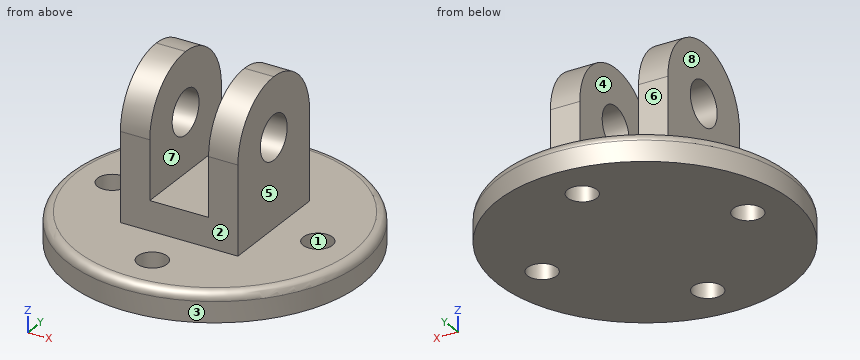
```python
from build123d import *

# Parameters (mm, degrees)
F0_R     = 63.5
F0_R_2   = 6.35
F1_DEPTH = 12.7
F2_R     = 3.81
F4_DEPTH = 25.4
F5_R     = 9.525
F6_DEPTH = 88.901


with BuildPart() as f1:
    # F0 (on Top) → F1 (new body)
    with BuildSketch(Plane.XY):
        Circle(F0_R)
        with Locations((0, -44.45)):
            Circle(F0_R_2, mode=Mode.SUBTRACT)
        with Locations((-44.45, 0)):
            Circle(F0_R_2, mode=Mode.SUBTRACT)
        with Locations((44.45, 0)):
            Circle(F0_R_2, mode=Mode.SUBTRACT)
        with Locations((0, 44.45)):
            Circle(F0_R_2, mode=Mode.SUBTRACT)
    extrude(amount=F1_DEPTH)

    # F2
    f2_edges = [f1.edges().sort_by_distance(p)[0] for p in [
        (-63.5, 0, 12.7),
    ]]
    fillet(f2_edges, radius=F2_R)

    # F3 (on Front) → F4 (join, symmetric)
    with BuildSketch(Plane.XZ):
        Polygon((-25.4, 76.2), (-25.4, 12.7), (25.4, 12.7), (25.4, 76.2), (12.7, 76.2), (12.7, 25.4), (-12.7, 25.4), (-12.7, 76.2), align=None)
    extrude(amount=F4_DEPTH, both=True)

    # F5 (on face) → F6 (cut, through all)
    with BuildSketch(Plane.YZ.offset(25.4)):
        with Locations((0, 50.8)):
            Circle(F5_R)
        with BuildLine():
            ThreePointArc((0, 76.2), (17.960512, 68.760512), (25.4, 50.8))
            Line((25.4, 50.8), (25.4, 76.2))
            Line((25.4, 76.2), (0, 76.2))
        make_face()
        with BuildLine():
            ThreePointArc((-25.4, 50.8), (-17.960512, 68.760512), (0, 76.2))
            Line((0, 76.2), (-25.4, 76.2))
            Line((-25.4, 76.2), (-25.4, 50.8))
        make_face()
    extrude(amount=-F6_DEPTH, mode=Mode.SUBTRACT)


solid = f1.part
```
Could you check a few things on this model? Use its own coordinates, in mm. Face numbers are marked on the shaded views. A direction names the side the tool comes from. Coordinates: 2 decimals unless noted, no trailing zeros. Loops run counter-clockwise (first coordinate to the right, second up) from the corner with the lowest first, then second, coordinate; pieces in that order, holes last. Notation, with made-up numbers: M 47,70.5 L 73,70.5 A18 cw 73,96.5 Z; hole C 24.25,-39.5 d10. An arc over 180 degrees is marked long. Put each result on its own line as item: value. Start each with the question number.
(1) Suppose I cut it at A-A on x = 0. Please give me the cut outline in (y, z), then the cut area to 3 significant figures.
(2) Thinking about a two-plate mould opening in X: for the marked faces 1, 2, 3 and 4, which applies, pulls with the +X half, pulls with the -X half, needs draft (parallel to the pull), parting line crosses it, or undercut?
(3) I need wall thicknesses on line 1 (Y direction, x = 0, z = 6.25); line 2 (X direction, y = 17, z = 17); line 3 (X direction, y = -3.5, z = 31.5). Which ranges of each line are inside material? Lowest first, please. Write a range as from..to.
(4) For the marked faces 5, 6, 7 and 8, which set-ups out of +Z, -Z, +X, -X, +Y, -Y let a thin tool reach every point of the face, with its end or its side?
(5) Will these pins go through, and if not, where does the flat tip stop? P1, Ø1, axis at x = -17, z = 63.5, coming from the -Y side; P2, Ø10, axis at x = 0, y = 44.45, coming from the +Z side; P3, Ø3, axis at x = -14, z = 15.5, coming from the +Y side; P4, Ø1, axis at y = -25.5, z = 44.5, coming from the +X side.
(6) Suppose I cut it at C-C on z = 62.5. Please give me the cut outline in (x, y), then the cut area to 3 significant figures.
(7) Suppose I cut it at B-B on z = 71. Please give me the cut outline in (x, y), then the cut area to 3 significant figures.
Solutions:
1. outline: M -63.5,0 L -50.8,0 L -50.8,12.7 L -59.69,12.7 A3.81 ccw -63.5,8.89 Z; M -38.1,0 L 38.1,0 L 38.1,12.7 L 25.4,12.7 L 25.4,25.4 L -25.4,25.4 L -25.4,12.7 L -38.1,12.7 Z; M 50.8,0 L 63.5,0 L 63.5,8.89 A3.81 ccw 59.69,12.7 L 50.8,12.7 Z
1. area: 1,930 mm2
2. face 1: undercut
2. face 2: needs draft
2. face 3: parting line crosses it
2. face 4: undercut
3. line 1: y = -63.5..-50.8, -38.1..38.1, 50.8..63.5
3. line 2: x = -25.4..25.4
3. line 3: x = -25.4..-12.7, 12.7..25.4
4. face 5: +Z, +X, +Y, -Y
4. face 6: +Z, +X, -X, +Y
4. face 7: +Z, +Y, -Y
4. face 8: +Z, -X, +Y, -Y
5. P1: stops at y = -22.28
5. P2: passes through
5. P3: stops at y = 25.4
5. P4: stops at x = 25.4
6. outline: M -25.4,-22.54 L -12.7,-22.54 L -12.7,22.54 L -25.4,22.54 Z; M 12.7,-22.54 L 25.4,-22.54 L 25.4,22.54 L 12.7,22.54 Z
6. area: 1,150 mm2
7. outline: M -25.4,-15.4 L -12.7,-15.4 L -12.7,15.4 L -25.4,15.4 Z; M 12.7,-15.4 L 25.4,-15.4 L 25.4,15.4 L 12.7,15.4 Z
7. area: 782 mm2
